For this review, take the finished solid that the model builds, in its own axes (mm). Face numbers are marked on the shaded views. A direction names the side the tool comes from. Round coordinates to 2 decimals unless told otherwise and drop trailing zeros. Order: outer loops, then holes, each group sorted by start corner. A loop starts at its lowest first (then second) coordinate and runs counter-clockwise, first axis right, second up. Notation, with made-up numbers: (34, 71.5) - (75, 71.5) arc R24 cw to (75, 99.5) - close; hole circle Ø2 at (31, -8.75). An arc over 180 degrees is marked (long way). One line per question, with ' | ' between items.
```python
from build123d import *

# Parameters (mm, degrees)
SKETCH_1_W          = 36
SKETCH_1_H          = 32
SKETCH_1_R          = 1.6
EXTRUDE_1_DEPTH     = 4
EXTRUDE_2_DEPTH     = 32
SKETCH_8_R          = 1.6
CUT_EXTRUDE_1_DEPTH = 53.619768148
SKETCH1_W           = 4
SKETCH1_H           = 32
BOSS_EXTRUDE1_DEPTH = 3
SKETCH2_W           = 5
SKETCH2_H           = 32
BOSS_EXTRUDE2_DEPTH = 12
CUT_EXTRUDE1_DEPTH  = 5
BOSS_EXTRUDE5_DEPTH = 5
BOSS_EXTRUDE6_START = 3
SKETCH7_W           = 15
SKETCH7_H           = 32
SKETCH7_R           = 1.6
BOSS_EXTRUDE6_DEPTH = 3
CUT_EXTRUDE2_DEPTH  = 0.25
BOSS_EXTRUDE7_START = 2.5
SKETCH9_W           = 15
SKETCH9_H           = 32
SKETCH9_R           = 1.6
BOSS_EXTRUDE7_DEPTH = 2.5
BOSS_EXTRUDE8_DEPTH = 2.5
CUT_EXTRUDE3_DEPTH  = 2.5
FILLET2_R           = 3
FILLET4_R           = 3
FILLET5_R           = 3
FILLET9_R           = 1
CUT_EXTRUDE4_DEPTH  = 3
CUT_EXTRUDE5_DEPTH  = 3
FILLET14_R          = 1
CHAMFER_1_SIZE      = 5
CHAMFER_1_SIZE2     = 2.886751346


with BuildPart() as part:
    # Эскиз1 → Бобышка-Вытянуть1 (new body)
    with BuildSketch(Plane.XY):
        with Locations((18, 16)):
            Rectangle(SKETCH_1_W, SKETCH_1_H)
        with Locations((8, 26)):
            Circle(SKETCH_1_R, mode=Mode.SUBTRACT)
        with Locations((28, 26)):
            Circle(SKETCH_1_R, mode=Mode.SUBTRACT)
        with Locations((8, 6)):
            Circle(SKETCH_1_R, mode=Mode.SUBTRACT)
        with Locations((28, 6)):
            Circle(SKETCH_1_R, mode=Mode.SUBTRACT)
    extrude(amount=EXTRUDE_1_DEPTH)

    # Эскиз7 → Бобышка-Вытянуть2 (add)
    with BuildSketch(Plane(origin=(0, 32, 0), x_dir=(1, 0, 0), z_dir=(0, 1, 0))):
        Polygon((0, 0), (-1.2, 0), (-1.2, 15), (-5.2, 15), (-5.2, -19), (-1.2, -19), (-1.2, -4), (0, -4), align=None)
    extrude(amount=-EXTRUDE_2_DEPTH)

    # Эскиз8 → Вырез-Вытянуть1 (cut, through all)
    with BuildSketch(Plane(origin=(-1.2, 0, 0), x_dir=(0, 0, -1), z_dir=(1, 0, 0))):
        with Locations(Location((8, 24, 0), (0, 0, 90))):
            Circle(SKETCH_8_R)
        with Locations(Location((8, 8, 0), (0, 0, 90))):
            Circle(SKETCH_8_R)
        with Locations(Location((-12, 8, 0), (0, 0, 90))):
            Circle(SKETCH_8_R)
        with Locations(Location((-12, 24, 0), (0, 0, 90))):
            Circle(SKETCH_8_R)
    extrude(amount=-CUT_EXTRUDE_1_DEPTH, mode=Mode.SUBTRACT)

    # Sketch1 → Boss-Extrude1 (add)
    with BuildSketch(Plane(origin=(36, 0, 0), x_dir=(0, 0, -1), z_dir=(1, 0, 0))):
        with Locations((-2, 16)):
            Rectangle(SKETCH1_W, SKETCH1_H)
    extrude(amount=BOSS_EXTRUDE1_DEPTH)

    # Sketch2 → Boss-Extrude2 (add)
    with BuildSketch(Plane(origin=(0, 0, 0), x_dir=(-1, 0, 0), z_dir=(0, 0, -1))):
        with Locations((-36.5, 16)):
            Rectangle(SKETCH2_W, SKETCH2_H)
    extrude(amount=BOSS_EXTRUDE2_DEPTH)

    # Sketch3 → Cut-Extrude1 (cut)
    with BuildSketch(Plane(origin=(39, 0, 0), x_dir=(0, 0, -1), z_dir=(1, 0, 0))):
        Polygon((7, 32), (12, 32), (12, 23.339745962), align=None)
        Polygon((12, 8.660254038), (7, 0), (12, 0), align=None)
    extrude(amount=-CUT_EXTRUDE1_DEPTH, mode=Mode.SUBTRACT)

    # Sketch6 → Boss-Extrude5 (add)
    with BuildSketch(Plane(origin=(39, 0, 0), x_dir=(0, 0, -1), z_dir=(1, 0, 0))):
        Polygon((-16, 8.660254038), (-11, 0), (-4, 0), (-4, 32), (-11, 32), (-16, 23.339745962), align=None)
    extrude(amount=-BOSS_EXTRUDE5_DEPTH)

    # Sketch7 → Boss-Extrude6 (add)
    # profile 1 of 2: a face of its own
    with BuildSketch(Plane(origin=(-1.2, 0, 0), x_dir=(0, 0, -1), z_dir=(1, 0, 0)).offset(BOSS_EXTRUDE6_START)):
        with Locations((7.5, 16)):
            Rectangle(SKETCH7_W, SKETCH7_H)
        with Locations(Location((8, 24, 0), (0, 0, 90))):
            Circle(SKETCH7_R, mode=Mode.SUBTRACT)
        with Locations(Location((8, 8, 0), (0, 0, 90))):
            Circle(SKETCH7_R, mode=Mode.SUBTRACT)
    # profile 2 of 2: a face of its own
    with BuildSketch(Plane(origin=(-1.2, 0, 0), x_dir=(0, 0, -1), z_dir=(1, 0, 0)).offset(BOSS_EXTRUDE6_START)):
        with Locations((-11.5, 16)):
            Rectangle(SKETCH7_W, SKETCH7_H)
        with Locations(Location((-12, 24, 0), (0, 0, 90))):
            Circle(SKETCH7_R, mode=Mode.SUBTRACT)
        with Locations(Location((-12, 8, 0), (0, 0, 90))):
            Circle(SKETCH7_R, mode=Mode.SUBTRACT)
    extrude(amount=-BOSS_EXTRUDE6_DEPTH)

    # Sketch8 → Cut-Extrude2 (cut)
    with BuildSketch(Plane.ZY.offset(-34)):
        Polygon((-12, 23.339745962), (-12, 8.660254038), (-7, 0), (0, 0), (0, 32), (-7, 32), align=None)
        Polygon((4, 32), (4, 0), (11, 0), (16, 8.660254038), (16, 23.339745962), (11, 32), align=None)
    extrude(amount=-CUT_EXTRUDE2_DEPTH, mode=Mode.SUBTRACT)

    # Sketch9 → Boss-Extrude7 (add)
    with BuildSketch(Plane(origin=(1.8, 0, 0), x_dir=(0, 0, -1), z_dir=(1, 0, 0)).offset(BOSS_EXTRUDE7_START)):
        with Locations((7.5, 16)):
            Rectangle(SKETCH9_W, SKETCH9_H)
        with Locations(Location((8, 24, 0), (0, 0, 90))):
            Circle(SKETCH9_R, mode=Mode.SUBTRACT)
        with Locations(Location((8, 8, 0), (0, 0, 90))):
            Circle(SKETCH9_R, mode=Mode.SUBTRACT)
    extrude(amount=-BOSS_EXTRUDE7_DEPTH)

    # Sketch10 → Boss-Extrude8 (add)
    with BuildSketch(Plane.ZY.offset(-34.25)):
        Polygon((-7, 32), (-12, 23.339745962), (-12, 8.660254038), (-7, 0), (0, 0), (0, 32), align=None)
    extrude(amount=BOSS_EXTRUDE8_DEPTH)

    # Sketch11 → Cut-Extrude3 (cut)
    with BuildSketch(Plane.ZY.offset(-31.75)):
        Polygon((-7, 32), (-12, 23.339745962), (-12, 8.660254038), (-7, 0), align=None)
    extrude(amount=-CUT_EXTRUDE3_DEPTH, mode=Mode.SUBTRACT)

    # Fillet2
    # the kernel refuses this fillet: 3 mm, written as the material it takes off along each edge
    with BuildSketch(Plane(origin=(31.75, -7.395099729, -7), x_dir=(1, 0, 0), z_dir=(0, 1, 0))) as fillet2_piece_1:
        with BuildLine():
            CenterArc((3, -2.958039892), FILLET2_R, 99.594068227, 80.405931773)
            Line((0, -2.958039892), (-0.06, -2.958039892))
            Line((-0.06, -2.958039892), (-0.06, 0))
            Line((-0.06, 0), (0, 0.06))
            ThreePointArc((0, 0.06), (1.25, 0.06), (2.49, 0.059160798))
            Line((2.49, 0.059160798), (2.5, 0))
        make_face()
    extrude(amount=46.790199458, mode=Mode.SUBTRACT)

    # Fillet4
    fillet4_edges = [part.edges().sort_by_distance(p)[0] for p in [
        (36.625, 32, -7),
        (36.625, 0, -7),
        (36.625, 8.660254038, -12),
        (36.625, 23.339745962, -12),
    ]]
    fillet(fillet4_edges, radius=FILLET4_R)

    # Fillet5
    fillet5_edges = [part.edges().sort_by_distance(p)[0] for p in [
        (36.625, 32, 11),
        (36.625, 23.339745962, 16),
        (36.625, 8.660254038, 16),
        (36.625, 0, 11),
    ]]
    fillet(fillet5_edges, radius=FILLET5_R)

    # Fillet9
    fillet9_edges = [part.edges().sort_by_distance(p)[0] for p in [
        (39, 4.732050808, -9.732050808),
        (39, 16, -12),
        (39, 27.267949192, -9.732050808),
        (39, 32, 2),
        (39, 31.598076211, -6.767949192),
        (39, 23.31235552, -11.897777479),
        (39, 8.68764448, -11.897777479),
        (39, 0.401923789, -6.767949192),
        (39, 4.732050808, 13.732050808),
        (39, 0, 2),
        (39, 27.267949192, 13.732050808),
        (39, 16, 16),
        (39, 31.598076211, 10.767949192),
        (39, 23.31235552, 15.897777479),
        (39, 8.68764448, 15.897777479),
        (39, 0.401923789, 10.767949192),
    ]]
    fillet(fillet9_edges, radius=FILLET9_R)

    # Sketch12 → Cut-Extrude4 (cut)
    with BuildSketch(Plane(origin=(4.3, 0, 0), x_dir=(0, 0, -1), z_dir=(1, 0, 0))):
        Polygon((6.354551733, 26.85), (4.709103466, 24), (6.354551733, 21.15), (9.645448267, 21.15), (11.290896534, 24), (9.645448267, 26.85), align=None)
        Polygon((6.354551733, 10.85), (4.709103466, 8), (6.354551733, 5.15), (9.645448267, 5.15), (11.290896534, 8), (9.645448267, 10.85), align=None)
    extrude(amount=-CUT_EXTRUDE4_DEPTH, mode=Mode.SUBTRACT)

    # Sketch13 → Cut-Extrude5 (cut)
    with BuildSketch(Plane(origin=(1.8, 0, 0), x_dir=(0, 0, -1), z_dir=(1, 0, 0))):
        Polygon((-15.290896534, 24), (-13.645448267, 21.15), (-10.354551733, 21.15), (-8.709103466, 24), (-10.354551733, 26.85), (-13.645448267, 26.85), align=None)
        Polygon((-15.290896534, 8), (-13.645448267, 5.15), (-10.354551733, 5.15), (-8.709103466, 8), (-10.354551733, 10.85), (-13.645448267, 10.85), align=None)
    extrude(amount=-CUT_EXTRUDE5_DEPTH, mode=Mode.SUBTRACT)

    # Fillet14
    fillet14_edges = [part.edges().sort_by_distance(p)[0] for p in [
        (4.3, 32, -7.5),
        (4.3, 0, -7.5),
        (4.3, 16, -15),
        (-5.2, 16, -15),
        (-5.2, 32, 2),
        (-5.2, 0, 2),
    ]]
    fillet(fillet14_edges, radius=FILLET14_R)

    # Фаска1
    chamfer_1_edges = [part.edges().sort_by_distance(p)[0] for p in [
        (1.8, 16, 19),
    ]]
    chamfer_1_side = [part.faces().sort_by_distance(p)[0] for p in [
        (-1.693709632, 16, 19),
    ]]
    chamfer(chamfer_1_edges, length=CHAMFER_1_SIZE, length2=CHAMFER_1_SIZE2, reference=chamfer_1_side[0])


solid = part.part
```
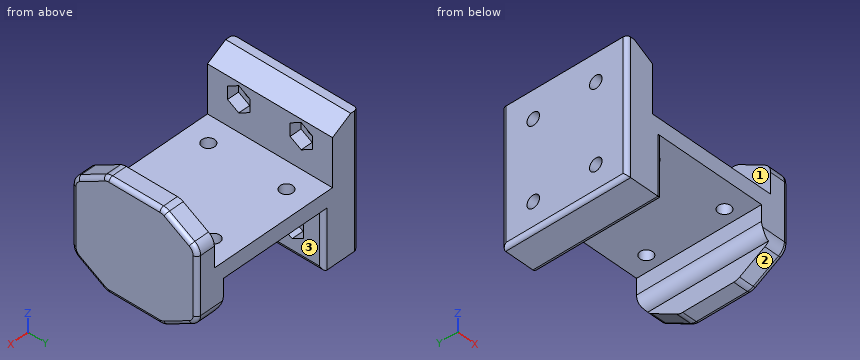
(1) We need section A-A on x = 28. State the section outline as (y, z) points.
Output values:
outline: (0, 0) - (4.4, 0) - (4.4, 4) - (0, 4) - close; (7.6, 0) - (24.4, 0) - (24.4, 4) - (7.6, 4) - close; (27.6, 0) - (32, 0) - (32, 4) - (27.6, 4) - close
(2) For probe 1 along Z at (x, y) = (-4, 24); probe 2 along Y at (x, z) = (28, 2); probe 3 along X at (y, z) = (20, -2), list the stretches that pass through material, from the lowest coordinate up. Write a range as [from, to].
Output values:
probe 1: [-15, -9.6], [-6.4, 10.4], [13.6, 19] | probe 2: [0, 4.4], [7.6, 24.4], [27.6, 32] | probe 3: [-5.2, 4.3], [31.75, 39]
(3) We need section B-B on z = 2.5. State the section outline as (x, y) points, plus the area to 3 significant figures.
Output values:
outline: (-5.2, 1) arc R1 ccw to (-4.2, 0) - (38, 0) arc R1 ccw to (39, 1) - (39, 31) arc R1 ccw to (38, 32) - (-4.2, 32) arc R1 ccw to (-5.2, 31) - close; hole circle Ø3.2 at (8, 6); hole circle Ø3.2 at (8, 26); hole circle Ø3.2 at (28, 6); hole circle Ø3.2 at (28, 26) | area: 1,380 mm^2
(4) For the marked faces 1, 2 and 3, list the 3-axis set-ups (+Z, -Z, +X, -X, +Y, -Y) from which the entire face can be reached by the end or side of a thin tool; tool diameter is ignored.
Output values:
face 1: +Z, +Y, -Y | face 2: -Z, +X, -Y | face 3: -Z, +Y, -Y
(5) We need section D-D on x = -2. State the section outline as (y, z) points, plus the area to 3 significant figures.
Output values:
outline: (0, -15) - (32, -15) - (32, 18.31) - (0, 18.31) - close; hole circle Ø3.2 at (8, -8); hole circle Ø3.2 at (8, 12); hole circle Ø3.2 at (24, -8); hole circle Ø3.2 at (24, 12) | area: 1,030 mm^2
(6) Insertion check: pin 1 (3.5 mm diameter, centred on x = 8, y = 6, fed in from -Z); pin 2 (16 mm diameter, centred on x = 14, y = 9.5, fed in from +Z); pin 3 (1.1 mm diameter, centred on x = 36.5, y = 16.5, fed in from +Z); pin 4 (5 mm diameter, centred on x = 4, z = 15, fed in from +Y). Each pin has a flat end and moves straight along its axis. Give the tip position at first contact, or say it passes through.
Output values:
pin 1: z = 0 | pin 2: z = 4 | pin 3: z = 16 | pin 4: y = 32
(7) We need section C-C on x = 35. State the section outline as (y, z) points, plus the area to 3 significant figures.
Output values:
outline: (0, -5.27) arc R3 ccw to (1.5, -7.87) - (7.96, -11.6) arc R3 ccw to (9.46, -12) - (22.54, -12) arc R3 ccw to (24.04, -11.6) - (30.5, -7.87) arc R3 ccw to (32, -5.27) - (32, 9.27) arc R3 ccw to (30.5, 11.87) - (24.04, 15.6) arc R3 ccw to (22.54, 16) - (9.46, 16) arc R3 ccw to (7.96, 15.6) - (1.5, 11.87) arc R3 ccw to (0, 9.27) - close | area: 807 mm^2
